Here's the drawing with two shaded views (mm, measured from the low corner). I have some questions. A direction names the side the tool comes from. Round coordinates to 2 decimals unless told otherwise and drop trailing zeros. Write each loop counter-clockwise with the first axis right and the second up, starting at its lowest first coordinate (ties: lowest second). Pieces come first, ordered by that corner, then holes. Notation, with made-up numbers: (84.25, -26) -> (114.25, -26) arc R19 ccw to (114.25, -4) -> close; hole circle Ø1 at (69.25, 42). An arc over 180 degrees is marked (long way). Use CSV: the item, a comma, the result in double quotes.
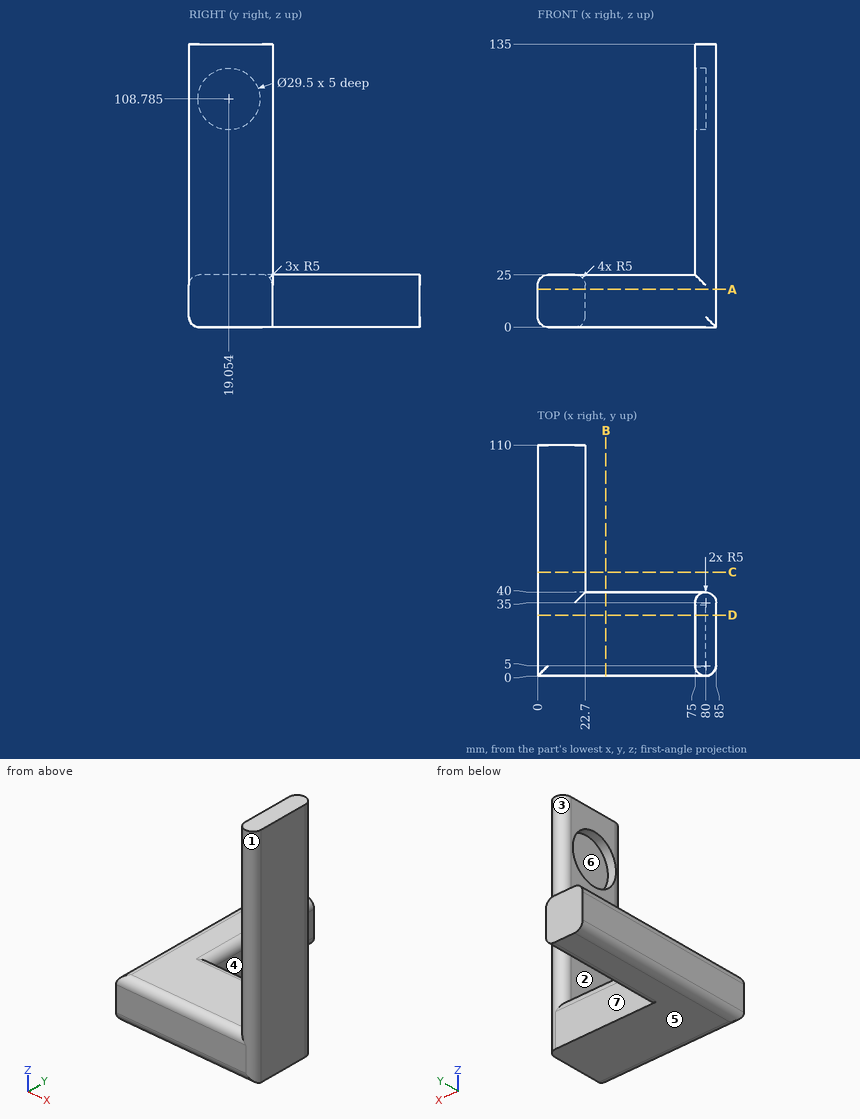
Q1. If we mould it in two halves opening along Y, with no side actions, what happens to the marked faces 5, 6 and 7? For each: released by +Y, released by -Y, zero draft, split by the parting line, or undercut.
Resolved:
face 5,"zero draft"
face 6,"undercut"
face 7,"released by +Y"
Q2. Please list where these lines run through material, in increasing order: probe 1 along Y at (x, z) = (79, 9); probe 2 along X at (y, z) = (11, 80); probe 3 along X at (y, z) = (10, 98).
Resolved:
probe 1,"y = 0 to 40"
probe 2,"x = 75 to 85"
probe 3,"x = 80 to 85"
Q3. Suppose I cut it at C-C (y = 49.5). Write out the boundary of the cut face in (x, z).
Resolved:
outline,"(0, 5) arc R5 ccw to (5, 0) -> (17.7, 0) arc R5 ccw to (22.7, 5) -> (22.7, 20) arc R5 ccw to (17.7, 25) -> (5, 25) arc R5 ccw to (0, 20) -> close"
Q4. Suppose I cut it at D-D (y = 29). Write out the boundary of the cut face in (x, z), and give its area (3 significant figures).
Resolved:
outline,"(0, 5) arc R5 ccw to (5, 0) -> (85, 0) -> (85, 135) -> (75, 135) -> (75, 119.68) -> (80, 119.68) -> (80, 97.89) -> (75, 97.89) -> (75, 25) -> (5, 25) arc R5 ccw to (0, 20) -> close"
area,"3,110 mm^2"
Q5. Will these pins go through, and if not, where does the flat tip stop? P1, Ø6, axis at x = 62.5, z = 5.5, coming from the +Y side; P2, Ø16.5, axis at y = 80.5, z = 9.5, coming from the +X side; P3, Ø9, axis at y = 19.5, z = 77.5, coming from the -X side.
Resolved:
P1,"stops at y = 40"
P2,"stops at x = 22.7"
P3,"stops at x = 75"
Q6. Suppose I cut it at A-A (z = 18). Write out the boundary of the cut face in (x, y).
Resolved:
outline,"(0, 0) -> (80, 0) arc R5 ccw to (85, 5) -> (85, 35) arc R5 ccw to (80, 40) -> (22.7, 40) -> (22.7, 110) -> (0, 110) -> close"
Q7. On a 3-axis mill with a long thin cutter (end or side, diameter ignored), from which of +Z, -Z, +X, -X, +Y, -Y can I reach the whole of each face in a straight line? I mean the marked faces 1, 2, 3 and 4. Say none if no direction works.
Resolved:
face 1,"+Z, -Y"
face 2,"+Z, -X, +Y, -Y"
face 3,"+Z, +Y"
face 4,"+Z, -Z, +X, +Y"
Q8. Suppose I cut it at B-B (x = 32.5). Write out the boundary of the cut face in (y, z), and give its area (3 significant figures).
Resolved:
outline,"(0, 5) arc R5 ccw to (5, 0) -> (40, 0) -> (40, 20) arc R5 ccw to (35, 25) -> (5, 25) arc R5 ccw to (0, 20) -> close"
area,"984 mm^2"
